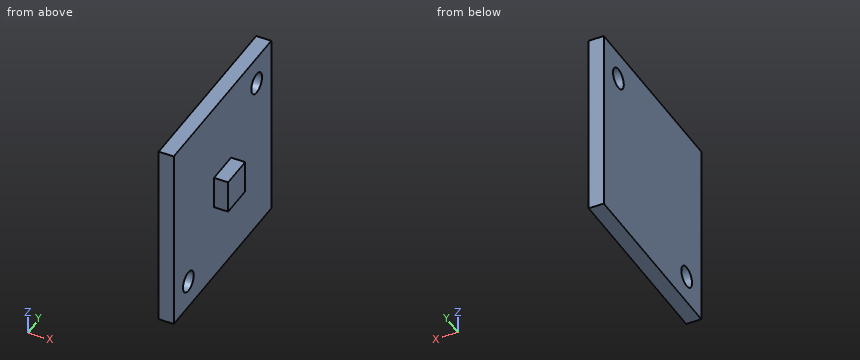
```python
from build123d import *

# Parameters (mm, degrees)
SKETCH1_W           = 20
SKETCH1_H           = 20
BOARD_DEPTH         = 1.6
SKETCH2_W           = 3.5
SKETCH2_H           = 3.5
UV_LED_3535_DEPTH   = 1.5
HOLES_M2_DEPTH      = 15.2323575
HOLES_M2_DEPTH_BACK = 15.2323575
SKETCH3_R           = 1.1


with BuildPart() as part:
    # Sketch1 → Board (new body)
    with BuildSketch(Plane(origin=(0, 0, 0), x_dir=(0, 0, -1), z_dir=(1, 0, 0))):
        Rectangle(SKETCH1_W, SKETCH1_H)
    extrude(amount=-BOARD_DEPTH)

    # Sketch2 → UV_LED_3535 (add)
    with BuildSketch(Plane(origin=(0, 0, 0), x_dir=(0, 0, -1), z_dir=(1, 0, 0))):
        Rectangle(SKETCH2_W, SKETCH2_H)
    extrude(amount=UV_LED_3535_DEPTH)

    # Sketch3 → Holes_M2 (cut, two sides: drawn at the far end of the back side and taken through both)
    with BuildSketch(Plane(origin=(0, 0, 0), x_dir=(0, 0, -1), z_dir=(1, 0, 0)).offset(-HOLES_M2_DEPTH_BACK)):
        with Locations(Location((7, -7, 0), (0, 0, 180))):
            Circle(SKETCH3_R)
        with Locations(Location((-7, 7, 0), (0, 0, 180))):
            Circle(SKETCH3_R)
    extrude(amount=HOLES_M2_DEPTH + HOLES_M2_DEPTH_BACK, mode=Mode.SUBTRACT)


solid = part.part
```
CAD build for the part. Positions are in the model's coordinates, mm. Give positions to 0.01 mm unless a question says otherwise; leave off trailing zeros. Loops run counter-clockwise (first coordinate to the right, second up) from the corner with the lowest first, then second, coordinate; pieces in that order, holes last. Notation, with made-up numbers: M -2,22.25 L 7,22.25 A24 cw 7,61.25 Z; hole C -16,-37.5 d5. An arc over 180 degrees is marked long. Use one line per item in the form item = value.
Item 1: Slice it at A-A (y = -7). List the corners of the cut face in (x, z).
Determined:
outline = M -1.6,-10 L 0,-10 L 0,-8.1 L -1.6,-8.1 Z; M -1.6,-5.9 L 0,-5.9 L 0,10 L -1.6,10 Z
Item 2: Slice it at D-D (x = -1.25). List the corners of the cut face in (y, z).
Determined:
outline = M -10,-10 L 10,-10 L 10,10 L -10,10 Z; hole C -7,-7 d2.2; hole C 7,7 d2.2
Item 3: Flat gauge pins, fed straight in: pin 1 (6 mm diameter, centred on y = 4.5, z = -1.5, fed in from +X); pin 2 (1.6 mm diameter, centred on x = 1, z = 0.5, fed in from -Y). Where does each tip first touch, or does it go through?
Determined:
pin_1 = 1.5
pin_2 = -1.75
Item 4: Slice it at B-B (z = 7). List the corners of the cut face in (x, y).
Determined:
outline = M -1.6,-10 L 0,-10 L 0,5.9 L -1.6,5.9 Z; M -1.6,8.1 L 0,8.1 L 0,10 L -1.6,10 Z
Item 5: Slice it at C-C (z = -0.5). List the corners of the cut face in (x, y).
Determined:
outline = M -1.6,-10 L 0,-10 L 0,-1.75 L 1.5,-1.75 L 1.5,1.75 L 0,1.75 L 0,10 L -1.6,10 Z
Item 6: Drill centre lines: probe 1 along Y at (x, z) = (-1.05, -7); probe 2 along Y at (x, z) = (-0.9, 7); probe 3 along X at (y, z) = (-9, -8.25). Where is each one in solid material? Low to high. Write a range as from..to.
Determined:
probe_1 = -10..-8.1, -5.9..10
probe_2 = -10..5.9, 8.1..10
probe_3 = -1.6..0
